Design review of the part built by this model. Coordinates are the model's own, in mm. A direction names the side the tool comes from. Coordinates: 2 decimals unless noted, no trailing zeros. Loops run counter-clockwise (first coordinate to the right, second up) from the corner with the lowest first, then second, coordinate; pieces in that order, holes last.
Q1. Machinability: for faces 1 (the face through (0, 6.35, 79)), 2 (the face through (-1.09, 1.7, 152.46)), which of the approach directions +Z, -Z, +X, -X, +Y, -Y give a long, thin tool a straight path to every point of the face, cutting with its end or side? Answer none if there is none.
Q2. Add section B-B on z = 49. Give the boundary of the cut face in (x, y).
Q3. For P1, Ø2.5, axis at x = 0, y = 0, coming from the +Z side; P2, Ø1, axis at y = 4, z = 90, coming from the +X side, all flat-tipped, find the tip position at first contact; note any pin that passes through.
Q4. Wall thickness on probe 1 along Y at (x, z) = (0, 136); probe 2 along Z at (x, y) = (-4.5, -3.5); probe 3 along X at (y, z) = (0, 148.5): over which ranges is each line inside the solid? List them lowest first.
Q5. Add section A-A on z = 126. Give the boundary of the cut face in (x, y).
Q6. Draft analysis for pull direction X (two halves, no side actions). For faces 3 (the face through (-5.474, 3.219, 78.89)), 4 (the face through (2, 2, 160.02)), 5 (the face through (1.239, -1.969, 144.356)), 6 (the face through (5.525, 3.131, 78.89)), state which applies: released by +X, released by -X, zero draft, split by the parting line, or undercut.
```python
from build123d import *

# Parameters (mm, degrees)
BOSS_EXTRUDE1_DEPTH        = 160.02
F_10_32_TAPPED_HOLE1_D     = 4.0386
F_10_32_TAPPED_HOLE1_DEPTH = 76.2
F_10_32_TAPPED_HOLE1_TIP   = 1.213317848
SKETCH5_R                  = 2.38125
CUT_EXTRUDE1_DEPTH         = 4.175
CUT_EXTRUDE1_DEPTH_BACK    = 16.875


with BuildPart() as part:
    # Sketch1 → Boss-Extrude1 (new body)
    with BuildSketch(Plane.XY):
        Polygon((7.332348419, 0), (3.666174209, 6.35), (-3.666174209, 6.35), (-7.332348419, 0), (-3.666174209, -6.35), (3.666174209, -6.35), align=None)
    extrude(amount=BOSS_EXTRUDE1_DEPTH)

    # #10-32 Tapped Hole1
    with Locations(Plane.XY.offset(160.02)):
        with Locations((0, 0)):
            Hole(F_10_32_TAPPED_HOLE1_D / 2, depth=F_10_32_TAPPED_HOLE1_DEPTH)
            with Locations((0, 0, -(F_10_32_TAPPED_HOLE1_DEPTH + F_10_32_TAPPED_HOLE1_TIP / 2))):  # 118° drill point
                Cone(0, F_10_32_TAPPED_HOLE1_D / 2, F_10_32_TAPPED_HOLE1_TIP, mode=Mode.SUBTRACT)

    # Sketch5 → Cut-Extrude1 (cut, two sides)
    with BuildSketch(Plane(origin=(5.499261314, 3.175, 0), x_dir=(0, 0, -1), z_dir=(0.866025404, 0.5, 0))) as cut_extrude1_sk:
        with Locations((-27.0002, 0)):
            Circle(SKETCH5_R)
        with Locations((-67.6402, 0)):
            Circle(SKETCH5_R)
        with Locations((-103.2002, 0)):
            Circle(SKETCH5_R)
        with Locations((-143.8402, 0)):
            Circle(SKETCH5_R)
    extrude(amount=CUT_EXTRUDE1_DEPTH, mode=Mode.SUBTRACT)
    extrude(cut_extrude1_sk.sketch, amount=-CUT_EXTRUDE1_DEPTH_BACK, mode=Mode.SUBTRACT)


solid = part.part
```
Entries:
1. face 1: +Z, -Z, +X, -X, +Y
1. face 2: +Z
2. outline: (-7.33, 0) - (-3.67, -6.35) - (3.67, -6.35) - (7.33, 0) - (3.67, 6.35) - (-3.67, 6.35) - close
3. P1: stops at z = 83.36
3. P2: stops at x = 5.31
4. probe 1: y = -6.35 to -2.02, 2.02 to 6.35
4. probe 2: z = 0 to 24.75, 29.25 to 65.39, 69.89 to 100.95, 105.45 to 141.59, 146.09 to 160.02
4. probe 3: x = -7.33 to -2.02, 2.02 to 7.33
5. outline: (-7.33, 0) - (-3.67, -6.35) - (3.67, -6.35) - (7.33, 0) - (3.67, 6.35) - (-3.67, 6.35) - close; hole circle Ø4.04 at (0, 0)
6. face 3: released by -X
6. face 4: zero draft
6. face 5: undercut
6. face 6: released by +X
